from build123d import *

# Parameters (mm, degrees)
F0_R     = 11.035
F2_DEPTH = 7
F3_SIZE  = 1
F4_COUNT = 3


with BuildPart() as f2:
    # F0 (on Top) → F2 (new body)
    with BuildSketch(Plane.XY):
        with BuildLine():
            ThreePointArc((-8, 12.729934), (-7.272249, -13.159241), (15.035, 0))
            ThreePointArc((15.035, 0), (13.159241, 7.272249), (8, 12.729934))
            ThreePointArc((8, 12.729934), (0, 15.035), (-8, 12.729934))
        make_face()
        Circle(F0_R, mode=Mode.SUBTRACT)
        Polygon((6.082385, 19.465), (12.16477, 30), (6.082385, 40.535), (-6.082385, 40.535), (-12.16477, 30), (-6.082385, 19.465), align=None)
        Polygon((7.545968, 30), (3.772984, 23.465), (-3.772984, 23.465), (-7.545968, 30), (-3.772984, 36.535), (3.772984, 36.535), align=None, mode=Mode.SUBTRACT)
        with BuildLine():
            ThreePointArc((-8, 12.729934), (0, 15.035), (8, 12.729934))
            Line((8, 12.729934), (18.247155, 19.465))
            Line((18.247155, 19.465), (12.16477, 30))
            Line((12.16477, 30), (6.082385, 19.465))
            Line((6.082385, 19.465), (-6.082385, 19.465))
            Line((-6.082385, 19.465), (-12.16477, 30))
            Line((-12.16477, 30), (-18.247155, 19.465))
            Line((-18.247155, 19.465), (-8, 12.729934))
        make_face()
    extrude(amount=F2_DEPTH)

    # F3
    f3_edges = [f2.edges().sort_by_distance(p)[0] for p in [
        (12.16477, 30, 7),
        (0, 40.535, 7),
        (-12.16477, 30, 0),
        (13.123578, 16.097467, 7),
        (-13.123578, 16.097467, 7),
        (13.123578, 16.097467, 0),
        (12.16477, 30, 0),
        (0, 40.535, 0),
        (-12.16477, 30, 7),
        (-7.272249, -13.159241, 0),
        (-7.272249, -13.159241, 7),
        (-13.123578, 16.097467, 0),
    ]]
    chamfer(f3_edges, length=F3_SIZE)

    # F4: F2 ×3 about axis
    f4_axis = Axis((0, 0, 32.696605), (0, 0, 1))


with BuildPart() as f2_1:
    add(f2.part)
    for i in range(1, F4_COUNT):
        add(f2.part.rotate(f4_axis, i * 360 / F4_COUNT))


solid = f2_1.part
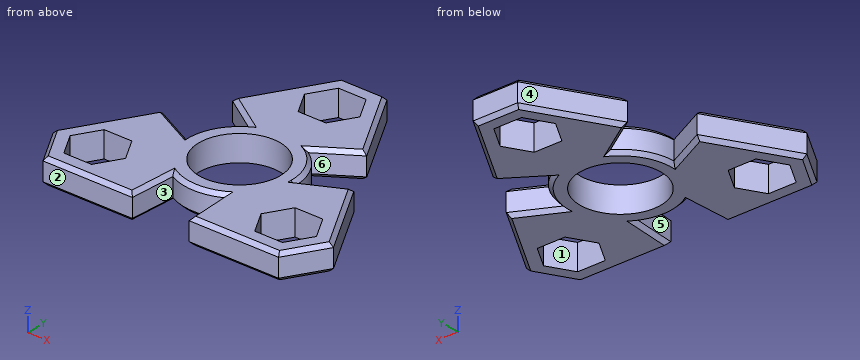
Read the model definition and answer for the solid it produces. Units are mm, in the model's axes. Face numbers are marked on the shaded views. A direction names the side the tool comes from. Give positions to 0.01 mm unless a question says otherwise; leave off trailing zeros. Write each loop counter-clockwise with the first axis right and the second up, starting at its lowest first coordinate (ties: lowest second). Pieces come first, ordered by that corner, then holes. Notation, with made-up numbers: (-20, 36.5) -> (27, 36.5) arc R32 cw to (27, 65.5) -> close; hole circle Ø3 at (-29.5, 48.5). An arc over 180 degrees is marked (long way). Answer as a JSON object with one key per item and string values. Group by question number.
1) The mould has two halves that part along Y. Classify the marked faces 4, 5 and 6: +Y half, -Y half, draft (parallel to the pull), parting line (faces both ways), or undercut.
2) Each of these flat-tipped pins is pushed along its axis until it touches: P1, Ø4, axis at y = -5, z = 1.5, coming from the +X side; P2, Ø2, axis at x = 0.5, z = 4.5, coming from the -Y side (3 decimals); P3, Ø4, axis at y = 7, z = 1, coming from the +X side; P4, Ø2, axis at x = -30, y = -16, coming from the -Z side. Where does it stop, or does it pass through?
3) Consider L1, parallel to Y at x = 0, z = 2.75 (3 decimals); L2, parallel to X at y = 0, z = 1.75 (3 decimals); L3, parallel to Y at x = 11.5, z = 3 (3 decimals). Determine where each line is inside the solid, lowest interval first. Write a range as from..to.
4) Find section A-A (x = 0). Write down the section's boundary in (y, z) (3 decimals).
5) Find section B-B (z = 2.5). Count the separate pieces of the cut face and the enclosed holes in it, and give its area (3 significant figures).
6) A tool of negligible diameter and unlimited length cuts with its end or side. For the marked faces 1, 2 and 3, from which of +Z, -Z, +X, -X, +Y, -Y can it reach the whole face along a straight path? Write none if from no direction.
7) Find section C-C (y = 16). Write down the section's boundary in (x, z), and give its area (3 significant figures).
Values follow:
{
 "1": {"face 4": "+Y half", "face 5": "-Y half", "face 6": "undercut"},
 "2": {"P1": "stops at x = 33.53", "P2": "stops at y = -15.035", "P3": "stops at x = 26.6", "P4": "passes through"},
 "3": {"L1": "y = -15.035..-11.035, 11.035..23.465, 36.535..40.535", "L2": "x = -29.485..-11.035, 11.035..29.485", "L3": "y = -25.535..9.685, 15.03..31.151"},
 "4": {"outline": "(-15.035, 1) -> (-14.035, 0) -> (-11.035, 0) -> (-11.035, 7) -> (-14.035, 7) -> (-15.035, 6) -> close; (11.035, 0) -> (23.465, 0) -> (23.465, 7) -> (11.035, 7) -> close; (36.535, 0) -> (39.535, 0) -> (40.535, 1) -> (40.535, 6) -> (39.535, 7) -> (36.535, 7) -> close"},
 "5": {"separate pieces": "1", "enclosed holes": "4", "area": "1,880 mm2"},
 "6": {"face 1": "+Z, -Z", "face 2": "+Z, -Z, +X, -X, -Y", "face 3": "+Z, -Z, -Y"},
 "7": {"outline": "(-12.98, 1) -> (-11.15, 0) -> (11.15, 0) -> (12.98, 1) -> (12.98, 6) -> (11.15, 7) -> (-11.15, 7) -> (-12.98, 6) -> close", "area": "178 mm2"}
}
